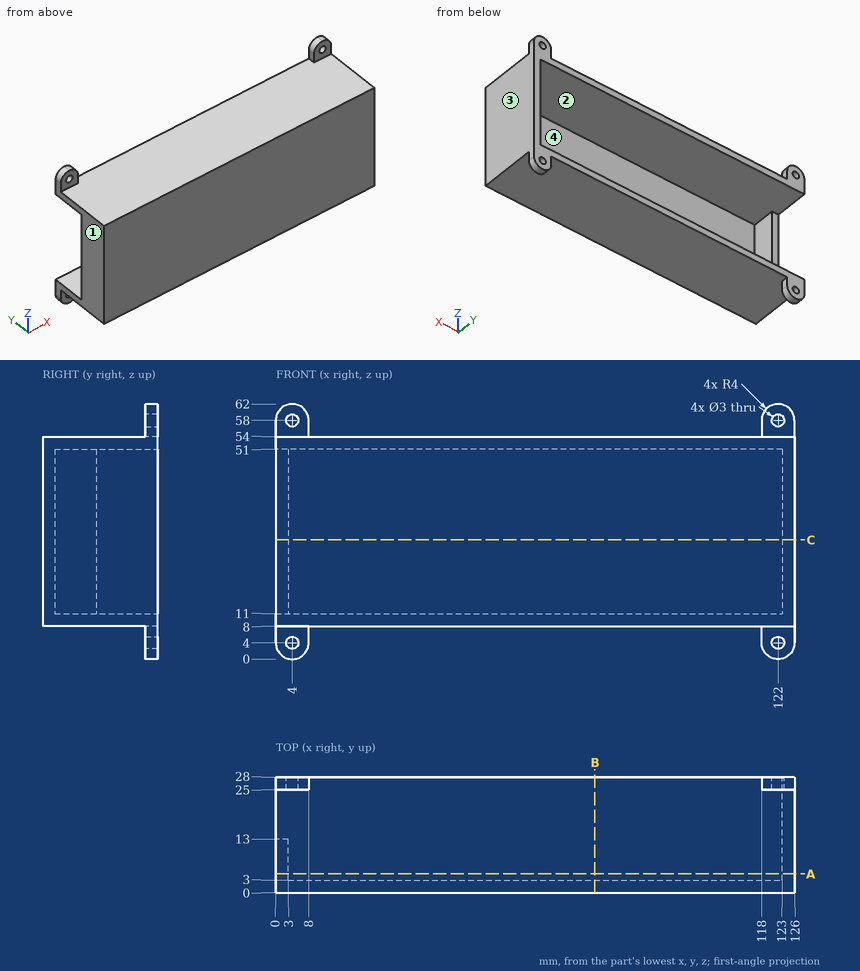
Answer from the drawing. Dimensions are ordinates in mm from the lowest x, y and z of the part. A direction names the side the tool comes from. Give positions to 0.01 mm unless a question says otherwise; leave off trailing zeros. Loops run counter-clockwise (first coordinate to the right, second up) from the corner with the lowest first, then second, coordinate; pieces in that order, holes last.
Item 1: For the marked faces 1 and 2, determine the directions among +Z, -Z, +X, -X, +Y, -Y from which every point of the face is accessible in a straight line to the end or side of a thin tool.
Item 2: The mould has two halves that part along Z. Classify the marked faces 3 and 4: released by +Z, released by -Z, zero draft, split by the parting line, or undercut.
Item 3: Each of these flat-tipped pins is pushed along its axis until it touches: pin 1 Ø3 at (y, z) = (9, 12) entering from -X; pin 2 Ø1.8 at (x, z) = (122, 58) entering from +Y; pin 3 Ø6.5 at (x, z) = (121.5, 58) entering from -Y; pin 4 Ø20 at (x, z) = (50, 25) entering from +Y. Where does it stop, or does it pass through?
Item 4: The part is cut by section B-B (x = 77.5). Write down the section's boundary in (y, z), and give its area (3 significant figures).
Item 5: Find the intervals of material crossed by line 1 along X through (y, z) = (27.1, 4); line 2 along Z through (x, y) = (122, 26.45); line 3 along Z through (x, y) = (104, 12.5), in increasing order.
Item 6: The part is cut by section A-A (y = 4.5). Write down the section's boundary in (x, z).
Item 7: The part is cut by section C-C (z = 29). Write down the section's boundary in (x, y).
Taken from the geometry:
1. face 1: +Z, -Z, -X, +Y, -Y
1. face 2: +Y
2. face 3: zero draft
2. face 4: undercut
3. pin 1: stops at x = 0
3. pin 2: passes through
3. pin 3: stops at y = 25
3. pin 4: stops at y = 3
4. outline: (0, 8) - (28, 8) - (28, 11) - (3, 11) - (3, 51) - (28, 51) - (28, 54) - (0, 54) - close
4. area: 288 mm2
5. line 1: x = 0 to 2.5, 5.5 to 8, 118 to 120.5, 123.5 to 126
5. line 2: z = 0 to 2.5, 5.5 to 11, 51 to 56.5, 59.5 to 62
5. line 3: z = 8 to 11, 51 to 54
6. outline: (0, 8) - (126, 8) - (126, 54) - (0, 54) - close; hole (3, 11) - (123, 11) - (123, 51) - (3, 51) - close
7. outline: (0, 0) - (126, 0) - (126, 28) - (123, 28) - (123, 3) - (3, 3) - (3, 13) - (0, 13) - close
